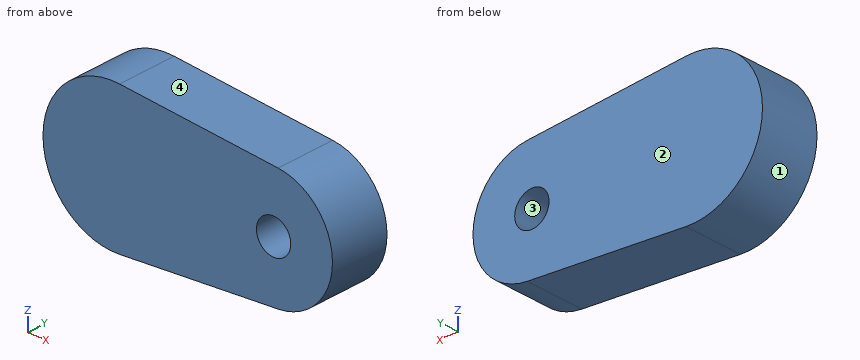
```python
from build123d import *

# Parameters (mm, degrees)
F0_R     = 1.75
F1_DEPTH = 3


with BuildPart() as f1:
    # F0 (on Front) → F1 (new body, symmetric)
    with BuildSketch(Plane.XZ):
        with BuildLine():
            Line((-15.692308, -7.228518), (0.461538, -5.982222))
            ThreePointArc((0.461538, -5.982222), (6, 0), (0.461538, 5.982222))
            Line((0.461538, 5.982222), (-15.692308, 7.228518))
            ThreePointArc((-15.692308, 7.228518), (-23.5, 0), (-15.692308, -7.228518))
        make_face()
        Circle(F0_R, mode=Mode.SUBTRACT)
    extrude(amount=F1_DEPTH, both=True)


solid = f1.part
```
Read the model definition and answer for the solid it produces. Units are mm, in the model's axes. Face numbers are marked on the shaded views. Give positions to 0.01 mm unless a question says otherwise; leave off trailing zeros. Write each loop counter-clockwise with the first axis right and the second up, starting at its lowest first coordinate (ties: lowest second). Pieces come first, ordered by that corner, then holes. Notation, with made-up numbers: M 4,64 L 46,64 A32 ccw 46,101 Z; hole C 16,-32 d3. An arc over 180 degrees is marked long. Put each result on its own line as item: value. Start each with the question number.
1. The part is cut by section B-B, the plane x = -0.5. Give the vertices of the cut face in (y, z), and give its area (3 significant figures).
2. The part is cut by section D-D, the plane x = -19.75. Give the vertices of the cut face in (y, z), and give its area (3 significant figures).
3. For a pull along Z with two mould halves and no side action, classify the marked faces 1, 2, 3 and 4 as released by +Z, released by -Z, zero draft, split by the parting line, or undercut.
4. Consider line 1 along Z through (x, y) = (0, 1.6); line 2 along Z through (x, y) = (-19, -2.15); line 3 along Z through (x, y) = (-19.5, -0.65). Determine where each line is inside the solid, lowest interval first.
5. Each of these flat-tipped pins is pushed along its axis until it touches: pin 1 Ø3 at (y, z) = (-0.5, -4.5) entering from +X; pin 2 Ø2 at (x, y) = (-4, 1) entering from -Z; pin 3 Ø1 at (x, y) = (-17.5, -0.5) entering from -Z. Where does it stop, or does it pass through?
6. The part is cut by section A-A, the plane y = -1.8. Give the vertices of the cut face in (x, z).
7. The part is cut by section C-C, the plane z = 5. Give the vertices of the cut face in (x, y), and give its area (3 significant figures).
Final values:
1. outline: M -3,-6.06 L 3,-6.06 L 3,-1.68 L -3,-1.68 Z; M -3,1.68 L 3,1.68 L 3,6.06 L -3,6.06 Z
1. area: 52.6 mm²
2. outline: M -3,-6.35 L 3,-6.35 L 3,6.35 L -3,6.35 Z
2. area: 76.2 mm²
3. face 1: split by the parting line
3. face 2: zero draft
3. face 3: undercut
3. face 4: released by +Z
4. line 1: z = -6.02 to -1.75, 1.75 to 6.02
4. line 2: z = -6.71 to 6.71
4. line 3: z = -6.48 to 6.48
5. pin 1: stops at x = 5.2
5. pin 2: stops at z = -6.4
5. pin 3: stops at z = -7.21
6. outline: M -15.69,-7.23 L 0.46,-5.98 A6 ccw 0.46,5.98 L -15.69,7.23 A7.25 ccw long Z; hole C 0,0 d3.5
7. outline: M -21.5,-3 L 3.32,-3 L 3.32,3 L -21.5,3 Z
7. area: 149 mm²
